from build123d import *

# Parameters (mm, degrees)
F0_R     = 165.1
F1_DEPTH = 12.7
F3_DEPTH = 25.4


with BuildPart() as f1:
    # F0 (on Top) → F1 (new body)
    with BuildSketch(Plane.XY):
        Circle(F0_R)
    extrude(amount=F1_DEPTH)

    # F2 (on face) → F3 (cut)
    with BuildSketch(Plane.XY.offset(12.7)):
        with BuildLine():
            Line((137.808496, -90.922101), (124.538028, -79.372378))
            Line((124.538028, -79.372378), (124.538028, -108.389527))
            ThreePointArc((124.538028, -108.389527), (131.463692, -99.876462), (137.808496, -90.922101))
        make_face()
        Polygon((124.538028, -108.389527), (124.538028, -79.372378), (110.168256, -95.883043), align=None)
        Polygon((110.168256, -95.883043), (99.283453, -108.389527), (124.538028, -108.389527), align=None)
        with BuildLine():
            Line((124.538028, -108.389527), (99.283453, -108.389527))
            Line((99.283453, -108.389527), (113.023665, -120.348083))
            ThreePointArc((113.023665, -120.348083), (118.931246, -114.513618), (124.538028, -108.389527))
        make_face()
        with BuildLine():
            Line((-99.283453, -108.389527), (-124.538028, -108.389527))
            ThreePointArc((-124.538028, -108.389527), (-118.931246, -114.513618), (-113.023665, -120.348083))
            Line((-113.023665, -120.348083), (-99.283453, -108.389527))
        make_face()
        Polygon((-110.168256, -95.883043), (-124.538028, -108.389527), (-99.283453, -108.389527), align=None)
        Polygon((-110.168256, -95.883043), (-124.538028, -79.372378), (-124.538028, -108.389527), align=None)
        with BuildLine():
            Line((-124.538028, -108.389527), (-124.538028, -79.372378))
            Line((-124.538028, -79.372378), (-137.808496, -90.922101))
            ThreePointArc((-137.808496, -90.922101), (-131.463692, -99.876462), (-124.538028, -108.389527))
        make_face()
        Polygon((-110.168256, 95.883043), (-124.538028, 108.389527), (-124.538028, 79.372378), align=None)
        with BuildLine():
            Line((-124.538028, 79.372378), (-124.538028, 108.389527))
            ThreePointArc((-124.538028, 108.389527), (-131.463692, 99.876462), (-137.808496, 90.922101))
            Line((-137.808496, 90.922101), (-124.538028, 79.372378))
        make_face()
        Polygon((-99.283453, 108.389527), (-124.538028, 108.389527), (-110.168256, 95.883043), align=None)
        with BuildLine():
            ThreePointArc((-113.023665, 120.348083), (-118.931246, 114.513618), (-124.538028, 108.389527))
            Line((-124.538028, 108.389527), (-99.283453, 108.389527))
            Line((-99.283453, 108.389527), (-113.023665, 120.348083))
        make_face()
        Polygon((124.538028, 108.389527), (99.283453, 108.389527), (110.168256, 95.883043), align=None)
        with BuildLine():
            Line((113.023665, 120.348083), (99.283453, 108.389527))
            Line((99.283453, 108.389527), (124.538028, 108.389527))
            ThreePointArc((124.538028, 108.389527), (118.931246, 114.513618), (113.023665, 120.348083))
        make_face()
        Polygon((124.538028, 79.372378), (124.538028, 108.389527), (110.168256, 95.883043), align=None)
        with BuildLine():
            ThreePointArc((137.808496, 90.922101), (131.463692, 99.876462), (124.538028, 108.389527))
            Line((124.538028, 108.389527), (124.538028, 79.372378))
            Line((124.538028, 79.372378), (137.808496, 90.922101))
        make_face()
    extrude(amount=-F3_DEPTH, mode=Mode.SUBTRACT)


solid = f1.part
Source: CAD feature listing. Evaluate the final solid. Frame: model axes, mm. A direction names the side the tool comes from. Give positions to 0.01 mm unless a question says otherwise; leave off trailing zeros. Write each loop counter-clockwise with the first axis right and the second up, starting at its lowest first coordinate (ties: lowest second). Pieces come first, ordered by that corner, then holes. Notation, with made-up numbers: M 31,68 L 76,68 A23 cw 76,87 Z; hole C -11,65.25 d5. An arc over 180 degrees is marked long. Return JSON: item names as keys, results as strings. Group by question number.
1) Pin query (flat end, axial travel): P1, Ø3, axis at x = 63, z = 3, coming from the -Y side; P2, Ø2, axis at y = 111, z = 8, coming from the +X side; P3, Ø1.5, axis at y = -29, z = 2.5, coming from the -X side. Return the tip coordinate at first contact, or that it passes through.
2) Cut plane A-A, the plane z = 5.75. Output: boundary loops of the cut face in (x, y), plus the area to 3 significant figures.
3) Cut plane C-C, the plane y = -50.5. Output: boundary loops of the cut face in (x, z).
4) Pull-direction query (Y, two-part tool) for faces 5 (the face through (131.27, -85.23, 6.44)), 6 (the face through (106.06, -114.29, 6.44)), 7 (the face through (1.74, 165.09, 6.26)); classes: pulls with the +Y half, pulls with the -Y half, needs draft (parallel to the pull), parting line crosses it, or undercut.
5) Material intervals for line 1 along Y through (x, z) = (-108, 9.5); line 2 along X through (y, z) = (-84.5, 3); line 3 along Y through (x, z) = (110, 10.5), sorted ascending. Write a range as [from, to].
6) Cut plane B-B, the plane x = 32.5. Output: boundary loops of the cut face in (y, z).
7) Set-up query: faces 1 (the face through (-131.27, 85.23, 6.44)), 2 (the face through (106.25, 114.453, 6.439)), 3 (the face through (-106.25, -114.453, 6.439)), 4 (the face through (-131.08, -85.066, 6.439)). Return all of +Z, -Z, +X, -X, +Y, -Y with unobstructed straight access to the full face (end or side cutting, diameter ignored); none if empty.
Recorded:
{
 "1": {"P1": "stops at y = -153.22", "P2": "stops at x = 103.43", "P3": "stops at x = -162.67"},
 "2": {"outline": "M -137.81,-90.92 L -124.54,-79.37 L -99.28,-108.39 L -113.02,-120.35 A165.1 ccw 113.02,-120.35 L 99.28,-108.39 L 124.54,-79.37 L 137.81,-90.92 A165.1 ccw 137.81,90.92 L 124.54,79.37 L 99.28,108.39 L 113.02,120.35 A165.1 ccw -113.02,120.35 L -99.28,108.39 L -124.54,79.37 L -137.81,90.92 A165.1 ccw Z", "area": "82,800 mm²"},
 "3": {"outline": "M -157.19,0 L 157.19,0 L 157.19,12.7 L -157.19,12.7 Z"},
 "4": {"face 5": "pulls with the -Y half", "face 6": "undercut", "face 7": "pulls with the +Y half"},
 "5": {"line 1": "y = [-124.88, -115.98], [-98.37, 98.37], [115.98, 124.88]", "line 2": "x = [-141.84, -130.43], [-120.08, 120.08], [130.43, 141.84]", "line 3": "y = [-123.12, -117.72], [-96.08, 96.08], [117.72, 123.12]"},
 "6": {"outline": "M -161.87,0 L 161.87,0 L 161.87,12.7 L -161.87,12.7 Z"},
 "7": {"face 1": "+Z, -Z, +Y", "face 2": "+Z, -Z, +X", "face 3": "+Z, -Z, -X", "face 4": "+Z, -Z, -Y"}
}
